from build123d import *

# Parameters (mm, degrees)
SKETCH_1_R        = 39.5
SKETCH_1_R_2      = 19
SKETCH_1_R_3      = 3
EXTRUDE_1_DEPTH   = 6
HOLE_WIZARD_M61_D = 6.4
CHAMFER_1_SIZE    = 0.5


with BuildPart() as part:
    # Эскиз1 → Вытянуть1 (new body)
    with BuildSketch(Plane(origin=(0, 0, 0), x_dir=(1, 0, 0), z_dir=(0, 1, 0))):
        Circle(SKETCH_1_R)
        Circle(SKETCH_1_R_2, mode=Mode.SUBTRACT)
        with Locations((0, 33.5)):
            Circle(SKETCH_1_R_3, mode=Mode.SUBTRACT)
        with Locations((33.5, 0)):
            Circle(SKETCH_1_R_3, mode=Mode.SUBTRACT)
        with Locations((-33.5, 0)):
            Circle(SKETCH_1_R_3, mode=Mode.SUBTRACT)
        with Locations((0, -33.5)):
            Circle(SKETCH_1_R_3, mode=Mode.SUBTRACT)
    extrude(amount=-EXTRUDE_1_DEPTH)

    # Отверстие с зазором M61 (through all)
    with Locations(Plane(origin=(0, 0, 0), x_dir=(-1, 0, 0), z_dir=(0, 1, 0))):
        with Locations((16.75, 29.011851027), (29.011851027, -16.75), (-16.75, -29.011851027), (-29.011851027, 16.75), (16.75, -29.011851027), (-29.011851027, -16.75), (-16.75, 29.011851027), (29.011851027, 16.75)):
            Hole(HOLE_WIZARD_M61_D / 2)

    # Фаска1
    chamfer_1_edges = [part.edges().sort_by_distance(p)[0] for p in [
        (-39.5, 0, 0),
        (-39.5, -6, 0),
    ]]
    chamfer(chamfer_1_edges, length=CHAMFER_1_SIZE)

    # Эскиз5 → Вырез-Повернуть1 (revolve, cut)
    with BuildSketch(Plane(origin=(0, 0, 0), x_dir=(1, 0, 0), z_dir=(0, 1, 0))):
        with BuildLine():
            Line((24.04163056, 24.04163056), (23.334523779, 23.334523779))
            ThreePointArc((23.334523779, 23.334523779), (23.334523779, 24.04163056), (24.04163056, 24.04163056))
        make_face()
    revolve(axis=Axis((26.47587554, 0, -26.47587554), (-0.707106781, 0, 0.707106781)), mode=Mode.SUBTRACT)


solid = part.part
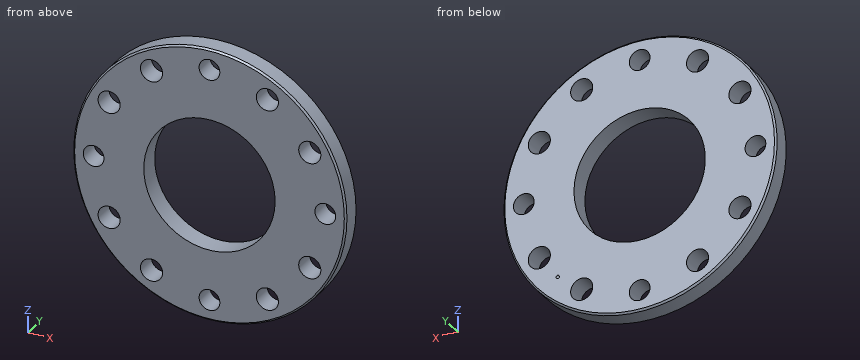
Verification items for the finished model (mm, model axes). Round coordinates to 2 decimals unless told otherwise and drop trailing zeros. Loops run counter-clockwise (first coordinate to the right, second up) from the corner with the lowest first, then second, coordinate; pieces in that order, holes last. Notation, with made-up numbers: (62, 42.25) - (76, 42.25) arc R14 cw to (76, 58.25) - close; hole circle Ø8 at (-38.75, 72.25). An arc over 180 degrees is marked (long way). Use a Markdown table: item, result. Add a question column.
1. Section check A-A, the plane z = 0. Record the boundary of the cut face in (x, y).
2. Section check B-B, the plane x = 0. Record the boundary of the cut face in (y, z).
3. Gauge pin test, flat ends, axial feed: pin 1 (3 mm diameter, centred on y = -3.5, z = -2.5, fed in from -X); pin 2 (5 mm diameter, centred on x = 33.5, z = 0, fed in from +Y); pin 3 (3 mm diameter, centred on x = -11.5, y = -5, fed in from -Z). Record the tip position at first contact, or that the pin passes through.
4. Section check C-C, the plane y = -3. Give the number of separate pieces and of enclosed holes in the cut face, plus the area to 3 significant figures.
5. Thickness scan on probe 1 along X at (y, z) = (-3.7, 0); probe 2 along X at (y, z) = (-1.95, -14.5). Record the ranges inside material, lowest first. Write a range as [from, to].
Checks:
| question | item | result |
|---|---|---|
| 1 | outline | (-39.5, -5.5) - (-39, -6) - (-36.5, -6) - (-36.5, 0) - (-39, 0) - (-39.5, -0.5) - close; (-30.5, -6) - (-19, -6) - (-19, 0) - (-30.5, 0) - close; (19, -6) - (30.5, -6) - (30.5, 0) - (19, 0) - close; (36.5, -6) - (39, -6) - (39.5, -5.5) - (39.5, -0.5) - (39, 0) - (36.5, 0) - close |
| 2 | outline | (-6, -39) - (-5.5, -39.5) - (-0.5, -39.5) - (0, -39) - (0, -36.5) - (-6, -36.5) - close; (-6, -30.5) - (0, -30.5) - (0, -19) - (-6, -19) - close; (-6, 19) - (0, 19) - (0, 30.5) - (-6, 30.5) - close; (-6, 36.5) - (0, 36.5) - (0, 39) - (-0.5, 39.5) - (-5.5, 39.5) - (-6, 39) - close |
| 3 | pin 1 | stops at x = -39.49 |
| 3 | pin 2 | passes through |
| 3 | pin 3 | stops at z = -38.21 |
| 4 | separate pieces | 1 |
| 4 | enclosed holes | 13 |
| 4 | area | 3,400 mm^2 |
| 5 | probe 1 | x = [-39.5, -36.5], [-30.5, -19], [19, 30.5], [36.5, 39.5] |
| 5 | probe 2 | x = [-36.74, -31.29], [-26.74, -12.28], [12.28, 26.74], [31.29, 36.74] |
